Autodesk Inventor part; units mm, degrees
ref_plane "YZ Plane" through (0, 0, 0) normal (1, 0, 0) x (0, 1, 0)
ref_plane "XZ Plane" through (0, 0, 0) normal (0, 1, 0) x (-1, 0, 0)
ref_plane "XY Plane" through (0, 0, 0) normal (0, 0, 1) x (1, 0, 0)
sketch "スケッチ1" plane through (0, 0, 0) normal (0, 0, 1) x (1, 0, 0)
  line L0 (-4, 25.75) -> (4, 25.75)
  line L1 (4, 25.75) -> (4, 17.5499)
  line L2 (-4, 17.5499) -> (-4, 25.75)
  line L3 (4, -17.5499) -> (4, -25.75)
  line L4 (4, -25.75) -> (-4, -25.75)
  line L5 (-4, -25.75) -> (-4, -17.5499)
  line L6 (0, -36.05) -> (0, 36.05)
  arc A0 (4, 17.5499) -> (-4, 17.5499) centre (0, 0) ccw
  arc A1 (-4, -17.5499) -> (4, -17.5499) centre (0, 0) ccw
  point P0 (0, 18)
  dimension "d1" = 18
  dimension "d2" = 18
  dimension "d3" = 51.5
  dimension "d4" = 25.75
  dimension "d5" = 8
extrude "押し出し1" add sketch "スケッチ1" along normal blind 5
chamfer "面取り1" distance 2 angle 45 2 edges at (0, 25.75, 5) (0, -25.75, 5)
sketch "スケッチ2" plane through (0, 0, 5) normal (0, 0, 1) x (1, 0, 0)
  line L0 (4, 25.75) -> (4, 17.5499)
  circle A0 centre (0, 0) radius 18
  circle A1 centre (0, 0) radius 19.25
  dimension "d15" = 38.5
extrude "押し出し2" add sketch "スケッチ2" along normal blind 7 and the other way blind 2
sketch "スケッチ3" plane through (0, 0, 3) normal (0, 0, -1) x (-1, 0, 0)
  line L0 (18.6548, 4.75) -> (20.5, 4.75)
  line L1 (20.5, 4.75) -> (20.5, -4.75)
  line L2 (20.5, -4.75) -> (18.6548, -4.75)
  arc A0 (4, -18.8298) -> (4, 18.8298) centre (0, 0) ccw
  line L3 (28.45, 0) -> (-27.2, 0)
  arc A1 (4, -17.5499) -> (4, 17.5499) centre (0, 0) ccw
  point P0 (20.5, 0)
  point P1 (18, 0)
  dimension "d16" = 9.5
  dimension "d17" = 2.5
extrude "押し出し3" add sketch "スケッチ3" against normal blind 1.8
chamfer "面取り2" distance 1.84 angle 45 2 edges at (-20.5, 4.75, 3.9) (-20.5, -4.75, 3.9)
sketch "スケッチ4" plane through (0, 0, 5) normal (0, 0, 1) x (1, 0, 0)
  circle A0 centre (0, 21.35) radius 1.35
  circle A1 centre (0, -21.35) radius 1.35
  line L0 (0, 20) -> (0, -20)
  point P0 (0, 0)
  point P1 (0, 0)
  dimension "d23" = 2.7
  dimension "d24" = 2.7
  dimension "d25" = 40
extrude "押し出し4" cut sketch "スケッチ4" against normal up to surface (5 mm away)
equation "\"d24\" = d23"
properties part number "conectcover"
Source: CAD feature listing. Evaluate the final solid. Frame: model axes, mm. A direction names the side the tool comes from. Round coordinates to 2 decimals unless told otherwise and drop trailing zeros. Loops run counter-clockwise (first coordinate to the right, second up) from the corner with the lowest first, then second, coordinate; pieces in that order, holes last.
1. Contact query for flat-ended pins moving along their axis: pin 1 (4 mm diameter, centred on y = -8, z = 9, fed in from +X); pin 2 (4 mm diameter, centred on y = -21, z = 3, fed in from +X); pin 3 (13 mm diameter, centred on x = -14, y = 7.5, fed in from -Z). Output: stop coordinate, or through.
2. Access query for faces 1 (the cylindrical face through (0, -18, 2)), 2 (the cylindrical face through (8.88, 17.08, 7.44)), 3 (the flat face through (13, -13, 12)). Directions: +Z, -Z, +X, -X, +Y, -Y. A direction counts if a zero-diameter tool reaches every point of the face in a straight line with its end or side. Return the directions, or none.
3. Ray query, L1, parallel to Y at x = 0, z = 1.3; L2, parallel to X at y = -21.35, z = 2.85; L3, parallel to X at y = 0.5, z = 4.25. Return the intervals inside material, ascending.
4. Section query B-B on x = -14. Output: boundary loops of the cut face in (y, z).
5. Section query A-A on y = 21.35. Output: boundary loops of the cut face in (x, z).
6. Section query C-C on y = 0. Output: boundary loops of the cut face in (x, z), and give its area (4 significant figures).
7. Section query D-D on z = 10.5. Output: boundary loops of the cut face in (x, y).
8. Mould query, pull axis X, two halves, no side actions, for faces 4 (the flat face through (-18.4, 0.1, 3)), 5 (the cylindrical face through (0.62, 20.15, 2.54)), 6 (the flat face through (-20.5, 0, 4)). Classes: released by +X, released by -X, zero draft, split by the parting line, or undercut.
Answers below:
1. pin 1: stops at x = 18.29
1. pin 2: stops at x = 4
1. pin 3: stops at z = 3
2. face 1: +Z, -Z
2. face 2: +Z
2. face 3: +Z, +X, -X, +Y, -Y
3. L1: y = -25.75 to -22.7, -20 to -18, 18 to 20, 22.7 to 25.75
3. L2: x = -4 to -1.35, 1.35 to 4
3. L3: x = -20.5 to -17.99, 17.99 to 19.24
4. outline: (-13.21, 3) - (-11.31, 3) - (-11.31, 12) - (-13.21, 12) - close; (11.31, 3) - (13.21, 3) - (13.21, 12) - (11.31, 12) - close
5. outline: (-4, 0) - (-1.35, 0) - (-1.35, 5) - (-4, 5) - close; (1.35, 0) - (4, 0) - (4, 5) - (1.35, 5) - close
6. outline: (-20.5, 3) - (-18, 3) - (-18, 12) - (-19.25, 12) - (-19.25, 4.8) - (-20.5, 4.8) - close; (18, 3) - (19.25, 3) - (19.25, 12) - (18, 12) - close
6. area: 24.75 mm2
7. outline: circle Ø38.5 at (0, 0); hole circle Ø36 at (0, 0)
8. face 4: zero draft
8. face 5: undercut
8. face 6: released by -X
